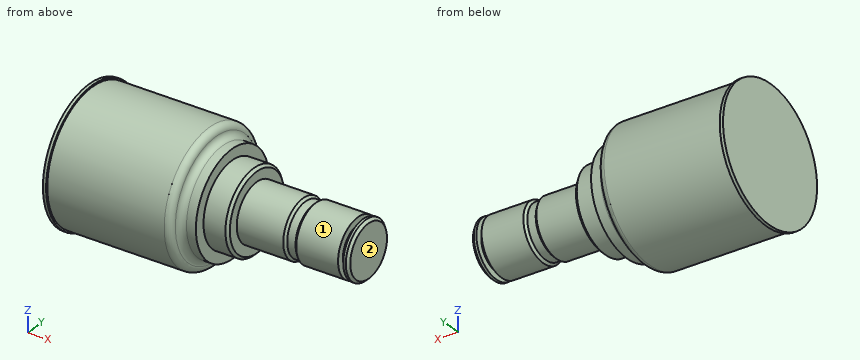
```python
from build123d import *

# Parameters (mm, degrees)
CHAMFER1_SIZE = 1.27


with BuildPart() as part:
    # Sketch1 → Revolve1 (revolve)
    with BuildSketch(Plane.XY):
        with BuildLine():
            Line((0, 0), (0, 32.5374))
            Line((0, 32.5374), (1.5748, 32.5374))
            Line((1.5748, 32.5374), (1.5748, 31.75))
            Line((1.5748, 31.75), (58.7248, 31.75))
            ThreePointArc((58.7248, 31.75), (60.991879668, 30.797830353), (61.899183307, 28.512425058))
            ThreePointArc((61.899183307, 28.512425058), (62.806486945, 26.227019762), (65.073566613, 25.274850115))
            Line((65.073566613, 25.274850115), (69.6468, 25.274850115))
            Line((69.6468, 25.274850115), (69.6468, 20.0025))
            Line((69.6468, 20.0025), (81.6356, 20.0025))
            Line((81.6356, 20.0025), (81.6356, 13.97))
            Line((81.6356, 13.97), (104.3686, 13.97))
            Line((104.3686, 13.97), (105.5116, 12.827))
            Line((105.5116, 12.827), (109.5756, 12.827))
            Line((109.5756, 12.827), (110.7186, 13.97))
            Line((110.7186, 13.97), (131.1656, 13.97))
            Line((131.1656, 13.97), (131.1656, 10.5918))
            Line((131.1656, 10.5918), (133.7056, 10.5918))
            Line((133.7056, 10.5918), (133.7056, 13.97))
            Line((133.7056, 13.97), (136.2456, 13.97))
            Line((136.2456, 13.97), (136.2456, 0))
            Line((136.2456, 0), (0, 0))
        make_face()
    revolve(axis=Axis((-9.339404577, 0, 0), (1, 0, 0)))

    # Chamfer1
    chamfer1_edges = [part.edges().sort_by_distance(p)[0] for p in [
        (81.6356, -20.0025, 0),
        (136.2456, -13.97, 0),
    ]]
    chamfer(chamfer1_edges, length=CHAMFER1_SIZE)


solid = part.part
```
Build history of the part. All positions in model axes, mm. Face numbers are marked on the shaded views. A direction names the side the tool comes from. Coordinates: 2 decimals unless noted, no trailing zeros. Write each loop counter-clockwise with the first axis right and the second up, starting at its lowest first coordinate (ties: lowest second). Pieces come first, ordered by that corner, then holes.
1. 3-axis set-ups, long thin cutter, end or side, ignore diameter. For the marked faces 1 and 2: which of +Z, -Z, +X, -X, +Y, -Y reach the whole face in a straight line?
Answer block:
face 1: +X
face 2: +Z, -Z, +X, +Y, -Y
2. Band-saw the part on A-A, the plane x = 36.5. Give the cut face in (y, z), and give its area (3 significant figures).
Answer block:
outline: circle Ø63.5 at (0, 0)
area: 3,170 mm2
3. Band-saw the part on B-B, the plane x = 72. Give the cut face in (y, z) (1 decimal), and give its area (3 significant figures).
Answer block:
outline: circle Ø40 at (0, 0)
area: 1,260 mm2
4. Drill centre lines: probe 1 along X at (y, z) = (-14.5, 28.5); probe 2 along X at (y, z) = (-7, -20.5); probe 3 along X at (y, z) = (-7.5, 10). Where is each one in solid material? Low to high.
Answer block:
probe 1: x = 0 to 1.57
probe 2: x = 0 to 69.65
probe 3: x = 0 to 131.17, 133.71 to 136.25
5. Drop flat-ended pins along their axis: pin 1 (8 mm diameter, centred on y = 14.5, z = 3, fed in from +X); pin 2 (12 mm diameter, centred on y = -24, z = 19.5, fed in from +X); pin 3 (6 mm diameter, centred on x = 64.5, z = 14.5, fed in from +Y); pin 4 (4 mm diameter, centred on x = 111.5, z = 2.5, fed in from -Y). Give the stop position or say it passes through.
Answer block:
pin 1: stops at x = 136.25
pin 2: stops at x = 69.65
pin 3: stops at y = 26.59
pin 4: stops at y = -13.96
